```python
from build123d import *

# Parameters (mm, degrees)
F0_R         = 14
F1_DEPTH     = 80
F3_R         = 18.5
F4_DEPTH     = 4
F8_DEPTH     = 4
F9_R         = 4.7
F10_R        = 2
F11_DEPTH    = 84.001
F12_R        = 10
F12_R_2      = 2
F13_DEPTH    = 70
F14_SIZE     = 1
F15_SIZE     = 0.5
F16_R        = 1.5
F17_DEPTH    = 25
F18_R        = 14
F18_R_2      = 12.5
F19_DEPTH    = 60
F20_S5_R     = 1.5
F20_T6_DEPTH = 28
F20_S7_R     = 18.5
F20_T8_DEPTH = 28


# Not quite as in the source:
# - a fillet or chamfer that OpenCascade refuses, or shapes differently, is made with other operations: its cross-section is extruded or revolved along the edge and cut away or added


with BuildPart() as f1:
    # F0 (on Top) → F1 (new body)
    with BuildSketch(Plane.XY):
        Circle(F0_R)
    extrude(amount=F1_DEPTH)

    # F3 (on offset) → F4 (join)
    with BuildSketch(Plane(origin=(0, 0, 20), x_dir=(1, 0, 0), z_dir=(0, 0, -1))):
        Circle(F3_R)
    extrude(amount=-F4_DEPTH)

    # F5 (on Front) → F6 (revolve, cut)
    with BuildSketch(Plane.XZ):
        Polygon((14, 15), (12, 13), (14, 11), align=None)
    revolve(axis=Axis((0, 0, 15.3274592012), (0, 0, 1)), mode=Mode.SUBTRACT)

    # F7 (on face) → F8 (join)
    with BuildSketch(Plane.XY.offset(80)):
        with BuildLine():
            Line((-3.3, -3.3), (-3.3, 0))
            Line((-3.3, 0), (-3.3, 3.3))
            Line((-3.3, 3.3), (-13.6055135882, 3.3))
            ThreePointArc((-13.6055135882, 3.3), (-14, 0), (-13.6055135882, -3.3))
            Line((-13.6055135882, -3.3), (-3.3, -3.3))
        make_face()
        Polygon((-3.3, 3.3), (-3.3, 0), (-3.3, -3.3), (0, -3.3), (3.3, -3.3), (3.3, 0), (3.3, 3.3), (0, 3.3), align=None)
        with BuildLine():
            Line((-3.3, 13.6055135882), (-3.3, 3.3))
            Line((-3.3, 3.3), (0, 3.3))
            Line((0, 3.3), (3.3, 3.3))
            Line((3.3, 3.3), (3.3, 13.6055135882))
            ThreePointArc((3.3, 13.6055135882), (0, 14), (-3.3, 13.6055135882))
        make_face()
        with BuildLine():
            Line((0, -3.3), (-3.3, -3.3))
            Line((-3.3, -3.3), (-3.3, -13.6055135882))
            ThreePointArc((-3.3, -13.6055135882), (0, -14), (3.3, -13.6055135882))
            Line((3.3, -13.6055135882), (3.3, -3.3))
            Line((3.3, -3.3), (0, -3.3))
        make_face()
        with BuildLine():
            Line((13.6055135882, 3.3), (3.3, 3.3))
            Line((3.3, 3.3), (3.3, 0))
            Line((3.3, 0), (3.3, -3.3))
            Line((3.3, -3.3), (13.6055135882, -3.3))
            ThreePointArc((13.6055135882, -3.3), (14, 0), (13.6055135882, 3.3))
        make_face()
    extrude(amount=F8_DEPTH)

    # F9
    f9_edges = [f1.edges().sort_by_distance(p)[0] for p in [
        (-3.3, 3.3, 82),
        (3.3, 3.3, 82),
        (3.3, -3.3, 82),
        (-3.3, -3.3, 82),
    ]]
    fillet(f9_edges, radius=F9_R)

    # F10 (on face) → F11 (cut, through all)
    with BuildSketch(Plane.XY.offset(84)):
        Circle(F10_R)
    extrude(amount=-F11_DEPTH, mode=Mode.SUBTRACT)

    # F12 (on face) + F8_face1 (on face) → F13 (cut)
    with BuildSketch(Plane(origin=(0, 0, 0), x_dir=(1, 0, 0), z_dir=(0, 0, -1))):
        Circle(F12_R)
        Circle(F12_R_2, mode=Mode.SUBTRACT)
        Circle(F12_R)
    with BuildSketch(Plane(origin=(-7.5775327369, -7.5775327369, 80), x_dir=(1, 0, 0), z_dir=(0, 0, 1))):
        with BuildLine():
            Line((-0.4224672631, 4.2775327369), (-6.0279808513, 4.2775327369))
            ThreePointArc((-6.0279808513, 4.2775327369), (-2.3219621997, -2.3219621997), (4.2775327369, -6.0279808513))
            Line((4.2775327369, -6.0279808513), (4.2775327369, -0.4224672631))
            ThreePointArc((4.2775327369, -0.4224672631), (2.9009346085, 2.9009346085), (-0.4224672631, 4.2775327369))
        make_face()
    extrude(amount=-F13_DEPTH, dir=(0, 0, -1), mode=Mode.SUBTRACT)

    # F14
    f14_edges = [f1.edges().sort_by_distance(p)[0] for p in [
        (-14, 0, 0),
    ]]
    chamfer(f14_edges, length=F14_SIZE)

    # F15
    f15_edges = [f1.edges().sort_by_distance(p)[0] for p in [
        (-18.5, 0, 20),
    ]]
    chamfer(f15_edges, length=F15_SIZE)

    # F16 (on face) → F17 (cut)
    with BuildSketch(Plane(origin=(0, 0, 20), x_dir=(1, 0, 0), z_dir=(0, 0, -1))):
        with Locations((11.4904851943, -11.4904851943)):
            Circle(F16_R)
    extrude(amount=-F17_DEPTH, mode=Mode.SUBTRACT)

    # F18 (on face) → F19 (cut, through all)
    with BuildSketch(Plane.XY.offset(84)):
        Circle(F18_R)
        Circle(F18_R_2, mode=Mode.SUBTRACT)
    extrude(amount=-F19_DEPTH, mode=Mode.SUBTRACT)

    # F20: chamfer of 6 on 1 edges, made by hand


with BuildPart() as f20_tool2:
    # F20_s3 → F20_t4 (revolve)
    with BuildSketch(Plane.XZ):
        Polygon((18.5, 24), (12.5, 30), (12.5, 24), align=None)
    revolve(axis=Axis((0, 0, 24), (0, 0, 1)))

    # F20_s5 → F20_t6 (cut, symmetric)
    with BuildSketch(Plane.XY.offset(27)):
        with Locations((11.4904851943, 11.4904851943)):
            Circle(F20_S5_R)
    extrude(amount=F20_T6_DEPTH, both=True, mode=Mode.SUBTRACT)

    # F20_s7 → F20_t8 (intersect, symmetric)
    with BuildSketch(Plane.XY.offset(27)):
        Circle(F20_S7_R)
    extrude(amount=F20_T8_DEPTH, both=True, mode=Mode.INTERSECT)


with BuildPart() as f1_1:
    add(f1.part)

    # F20_t1: union F20_tool2
    add(f20_tool2.part)


solid = f1_1.part
```
Work out the finished part from the listing and answer in its coordinate system (mm). A direction names the side the tool comes from. Round coordinates to 2 decimals unless told otherwise and drop trailing zeros. Loops run counter-clockwise (first coordinate to the right, second up) from the corner with the lowest first, then second, coordinate; pieces in that order, holes last. Notation, with made-up numbers: (23, -30) -> (70, -30) arc R31 cw to (70, -1) -> close; hole circle Ø5 at (29, 88). An arc over 180 degrees is marked (long way). Write each question's results on one line, items separated by ' | '. Start each with the question number.
1. Section D-D (z = 10) is taken. Determine the outline of the cut face in (x, y), plus the area to 3 significant figures.
2. A tool of negligible diameter and unlimited length cuts with its end or side. For faces 5 (the face through (3.3, 10, 82)), 6 (the face through (10, -3.3, 82)), 7 (the face through (9, 11, 20)), 8 (the face through (-4.713, -4.64, 82.028)), from which of +Z, -Z, +X, -X, +Y, -Y can it reach the whole face along a straight path? Write none if from no direction.
3. For a pull along X with two mould halves and no side action, classify faces 1 (the face through (12.932, -5.362, 5.93)), 2 (the face through (-7, 7, 80)), 3 (the face through (-0.1, -2.4, 70)), 4 (the face through (4.64, -4.713, 82.028)) as +X half, -X half, draft (parallel to the pull), parting line (faces both ways), or undercut.
4. Given pin 1 Ø5 at (x, z) = (6, 64) entering from +Y; pin 2 Ø2 at (x, z) = (-10.5, 82.5) entering from +Y; pin 3 Ø5 at (y, z) = (-12, 53) entering from +X; pin 4 Ø1 at (x, z) = (-13.5, 62.5) entering from +Y, each flat-ended and moving along its own axis, determine where each tip first touches the part or whether it passes through.
5. Find the intervals of material crossed by probe 1 along Y at (x, z) = (0, 73); probe 2 along X at (y, z) = (0, 22); probe 3 along Z at (x, y) = (8.5, -5), in increasing order. Write a range as from..to.
6. Section C-C (z = 78) is taken. Determine the outline of the cut face in (x, y), plus the area to 3 significant figures.
Evaluation:
1) outline: circle Ø28 at (0, 0); hole circle Ø20 at (0, 0) | area: 302 mm2
2) face 5: +Z, +X, +Y | face 6: +Z, +X, -Y | face 7: -Z | face 8: +Z, -X, -Y
3) face 1: parting line | face 2: draft | face 3: undercut | face 4: +X half
4) pin 1: stops at y = 12 | pin 2: stops at y = 3.3 | pin 3: stops at x = 8.12 | pin 4: passes through
5) probe 1: y = -12.5..-2, 2..12.5 | probe 2: x = -18.5..-10, 10..18.5 | probe 3: z = 70..80
6) outline: circle Ø25 at (0, 0); hole circle Ø4 at (0, 0) | area: 478 mm2
